```python
from build123d import *

# Parameters (mm, degrees)
F0_R      = 42.5
F1_DEPTH  = 15
F3_DEPTH  = 30
F2_R      = 22.5
F4_DEPTH  = 3
F5_R      = 10
F6_DEPTH  = 30
F7_DEPTH  = 15
F8_R      = 10
F9_DEPTH  = 30
F11_DEPTH = 220


with BuildPart() as f1:
    # F0 (on Top) → F1 (new body)
    with BuildSketch(Plane.XY):
        Circle(F0_R)
    extrude(amount=F1_DEPTH)

    # F2 (on Top) → F3 (join)
    with BuildSketch(Plane.XY):
        Polygon((223.814484, 47.5), (-76.185516, 47.5), (-76.185516, -92.5), (-56.101405, -92.5), (-56.101405, -22.5), (-31.101405, -22.5), (-31.101405, 33.5), (31.898595, 33.5), (31.898595, -22.5), (61.898595, -22.5), (61.898595, -92.5), (223.814484, -92.5), align=None)
    extrude(amount=-F3_DEPTH)

    # F2 (on Top) → F4 (join)
    with BuildSketch(Plane.XY):
        Polygon((223.814484, 47.5), (-76.185516, 47.5), (-76.185516, -92.5), (-56.101405, -92.5), (-56.101405, -22.5), (-31.101405, -22.5), (-31.101405, 33.5), (31.898595, 33.5), (31.898595, -22.5), (61.898595, -22.5), (61.898595, -92.5), (223.814484, -92.5), align=None)
        with BuildLine():
            Line((-56.101405, -22.5), (-56.101405, -92.5))
            Line((-56.101405, -92.5), (-43.213305, -92.5))
            ThreePointArc((-43.213305, -92.5), (-6.340398, -35.394619), (45, -79.945706))
            ThreePointArc((45, -79.945706), (44.551087, -86.286104), (43.213305, -92.5))
            Line((43.213305, -92.5), (61.898595, -92.5))
            Line((61.898595, -92.5), (61.898595, -22.5))
            Line((61.898595, -22.5), (31.898595, -22.5))
            Line((31.898595, -22.5), (31.898595, 33.5))
            Line((31.898595, 33.5), (-31.101405, 33.5))
            Line((-31.101405, 33.5), (-31.101405, -22.5))
            Line((-31.101405, -22.5), (-56.101405, -22.5))
        make_face()
        Circle(F2_R, mode=Mode.SUBTRACT)
        with BuildLine():
            ThreePointArc((45, -79.945706), (-6.340398, -35.394619), (-43.213305, -92.5))
            ThreePointArc((-43.213305, -92.5), (0, -124.945706), (43.213305, -92.5))
            ThreePointArc((43.213305, -92.5), (44.551087, -86.286104), (45, -79.945706))
        make_face()
    extrude(amount=F4_DEPTH)

    # F5 (on Top) → F6 (join)
    with BuildSketch(Plane.XY):
        Circle(F5_R)
    extrude(amount=-F6_DEPTH)

    # F5 (on Top) → F7 (join)
    with BuildSketch(Plane.XY):
        Circle(F5_R)
    extrude(amount=F7_DEPTH)

    # F8 (on Top) → F9 (join)
    with BuildSketch(Plane.XY):
        with Locations((0, -80.542963)):
            Circle(F8_R)
    extrude(amount=-F9_DEPTH)

    # F10 (on face) → F11 (join)
    with BuildSketch(Plane.XY.offset(15)):
        Polygon((-6, 27), (-6, 15), (0, 15), (6, 15), (6, 27), align=None)
        Polygon((6, -15), (0, -15), (-6, -15), (-6, -27), (6, -27), align=None)
    extrude(amount=F11_DEPTH)


solid = f1.part
```
Read the model definition and answer for the solid it produces. Units are mm, in the model's axes. A direction names the side the tool comes from. Give positions to 0.01 mm unless a question says otherwise; leave off trailing zeros. Write each loop counter-clockwise with the first axis right and the second up, starting at its lowest first coordinate (ties: lowest second). Pieces come first, ordered by that corner, then holes. Notation, with made-up numbers: (-23.5, -28) -> (23.5, -28) arc R13 cw to (23.5, -13) -> close; hole circle Ø2 at (26.5, -22). An arc over 180 degrees is marked (long way). Answer in a Markdown table with one row per item.
1) Section A-A on z = 119 is taken. Give the vertices of the cut face in (x, y), plus the area to 3 significant figures.
Results list:
| item | result |
|---|---|
| outline | (-6, -27) -> (6, -27) -> (6, -15) -> (-6, -15) -> close; (-6, 15) -> (6, 15) -> (6, 27) -> (-6, 27) -> close |
| area | 288 mm^2 |
2) Section C-C on x = 1 is taken. Give the vertices of the cut face in (y, z), plus the area to 3 significant figures.
Results list:
| item | result |
|---|---|
| outline | (-124.93, 0) -> (-90.49, 0) -> (-90.49, -30) -> (-70.59, -30) -> (-70.59, 0) -> (-9.95, 0) -> (-9.95, -30) -> (9.95, -30) -> (9.95, 0) -> (33.5, 0) -> (33.5, -30) -> (47.5, -30) -> (47.5, 3) -> (42.49, 3) -> (42.49, 15) -> (27, 15) -> (27, 235) -> (15, 235) -> (15, 15) -> (-15, 15) -> (-15, 235) -> (-27, 235) -> (-27, 15) -> (-42.49, 15) -> (-42.49, 3) -> (-124.93, 3) -> close |
| area | 8,430 mm^2 |
3) Section B-B on y = -38.5 is taken. Give the vertices of the cut face in (x, z), plus the area to 3 significant figures.
Results list:
| item | result |
|---|---|
| outline | (-76.19, -30) -> (-56.1, -30) -> (-56.1, 0) -> (61.9, 0) -> (61.9, -30) -> (223.81, -30) -> (223.81, 3) -> (18, 3) -> (18, 15) -> (-18, 15) -> (-18, 3) -> (-76.19, 3) -> close |
| area | 6,790 mm^2 |
4) Section D-D on y = 0 is taken. Give the vertices of the cut face in (x, z).
Results list:
| item | result |
|---|---|
| outline | (-76.19, -30) -> (-31.1, -30) -> (-31.1, 0) -> (-10, 0) -> (-10, -30) -> (10, -30) -> (10, 0) -> (31.9, 0) -> (31.9, -30) -> (223.81, -30) -> (223.81, 3) -> (42.5, 3) -> (42.5, 15) -> (-42.5, 15) -> (-42.5, 3) -> (-76.19, 3) -> close |
5) Determine the mould class of faces 5 (the flat face through (-64, -92.5, -14)), 6 (the cylindrical face through (-33.727, -25.861, 8.916)), 7 (the flat face through (0, -21, 235)), 8 (the cylindrical face through (4.614, -89.415, -14.79)) for opening direction Y: released by +Y, released by -Y, zero draft, split by the parting line, or undercut.
Results list:
| item | result |
|---|---|
| face 5 | released by -Y |
| face 6 | split by the parting line |
| face 7 | zero draft |
| face 8 | undercut |
6) Each of these flat-tipped pins is pushed along its axis until it touches: pin 1 Ø3.5 at (y, z) = (21.5, 144.5) entering from -X; pin 2 Ø13 at (y, z) = (-22, 141.5) entering from +X; pin 3 Ø13 at (x, z) = (-2, 126.5) entering from +Y; pin 4 Ø24 at (x, z) = (5.5, -8.5) entering from -Y. Where does it stop, or does it pass through?
Results list:
| item | result |
|---|---|
| pin 1 | x = -6 |
| pin 2 | x = 6 |
| pin 3 | y = 27 |
| pin 4 | y = -124.95 |
7) A tool of negligible diameter and unlimited length cuts with its end or side. For faces 1 (the flat face through (0, 27, 123)), 2 (the flat face through (6, 21, 123)), 3 (the flat face through (-6, -21, 123)), 4 (the flat face through (47, -22.5, -15)), from which of +Z, -Z, +X, -X, +Y, -Y can it reach the whole face along a straight path? Write none if from no direction.
Results list:
| item | result |
|---|---|
| face 1 | +Z, +X, -X, +Y |
| face 2 | +Z, +X, +Y, -Y |
| face 3 | +Z, -X, +Y, -Y |
| face 4 | -Z, -Y |
8) Straight lines are drawn through the part: line 1 (Y direction, x = -0.5, z = 143); line 2 (Z direction, x = -6, y = 34.5); line 3 (Z direction, x = 72, y = -19.5). For each, find the intervals that lie inside material, in ascending order. Write a range as [from, to].
Results list:
| item | result |
|---|---|
| line 1 | [-27, -15], [15, 27] |
| line 2 | [-30, 15] |
| line 3 | [-30, 3] |
